The listing builds one solid part. Answer for the finished solid, in the listing's coordinates (mm). Coordinates: 2 decimals unless noted, no trailing zeros. Loops run counter-clockwise (first coordinate to the right, second up) from the corner with the lowest first, then second, coordinate; pieces in that order, holes last. Notation, with made-up numbers: M 15,-14 L 53,-14 A13 ccw 53,-2 Z; hole C 85,32 d8. An arc over 180 degrees is marked long. Answer as a JSON object with one key per item and string values. Group by question number.
1. A cutting plane is placed at A-A on z = 40.5. Give the vertices of the cut face in (x, y).
2. Given pin 1 (7.5 mm diameter, centred on x = -261, z = -17.5, fed in from -Y); pin 2 (7.5 mm diameter, centred on x = 259, z = 12.5, fed in from +Y); pin 3 (12 mm diameter, centred on x = 254, y = -3.5, fed in from -Z); pin 4 (7.5 mm diameter, centred on x = -257.5, y = -3.5, fed in from +Z), each flat-ended and moving along its own axis, determine where each tip first touches the part or whether it passes through.
3. A straight line is drawn through the part: L1, parallel to X at y = 3.5, z = -41. Find the intervals that lie inside material, in ascending order.
from build123d import *

# Parameters (mm, degrees)
F0_W     = 20
F0_H     = 95
F1_DEPTH = 250
F2_W     = 15
F2_H     = 70
F3_DEPTH = 15


# Not quite as in the source:
# - a pattern or mirror of a feature is missing from the dataset's text; its kind, count and spacing are read off the source's solid


with BuildPart() as f1:
    # F0 (on Right) → F1 (new body, symmetric)
    with BuildSketch(Plane.YZ):
        Rectangle(F0_W, F0_H)
    extrude(amount=F1_DEPTH, both=True)

    # F2 (on face) → F3 (join)
    with BuildSketch(Plane.YZ.offset(250)):
        Rectangle(F2_W, F2_H)
    f3 = extrude(amount=F3_DEPTH)

    # F3_copies: F3 across plane
    add(f3.mirror(Plane(origin=(0, 0, 0), x_dir=(0, 0, -1), z_dir=(-1, 0, 0))))


solid = f1.part
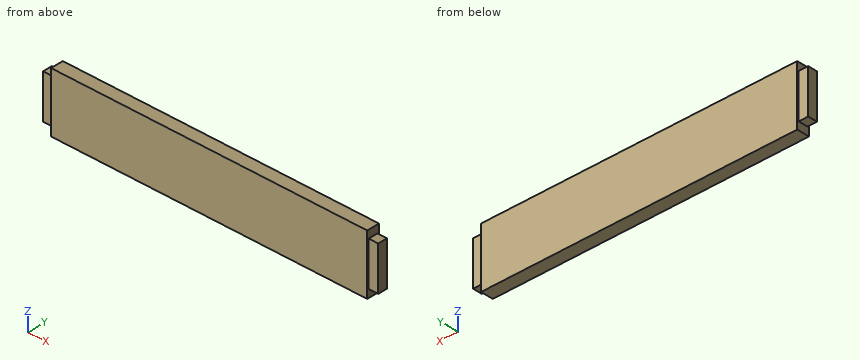
From the geometry:
{
 "1": {"outline": "M -250,-10 L 250,-10 L 250,10 L -250,10 Z"},
 "2": {"pin 1": "stops at y = -7.5", "pin 2": "stops at y = 7.5", "pin 3": "stops at z = -47.5", "pin 4": "stops at z = 35"},
 "3": {"L1": "x = -250 to 250"}
}
